For this review, take the finished solid that the model builds, in its own axes (mm). Face numbers are marked on the shaded views. A direction names the side the tool comes from. Coordinates: 2 decimals unless noted, no trailing zeros. Loops run counter-clockwise (first coordinate to the right, second up) from the corner with the lowest first, then second, coordinate; pieces in that order, holes last. Notation, with made-up numbers: M -29,36.25 L -15,36.25 A14 cw -15,53.25 Z; hole C -14.75,73.5 d6. An arc over 180 degrees is marked long. Answer as a JSON object with one key per item and string values. Group by question number.
Item 1: Add section A-A (y = -34.5). State the section outline as (x, z) points, then the cut area to 3 significant figures.
Item 2: Wall thickness on L1, parallel to X at y = -56, z = 38; L2, parallel to Z at x = 57.15, y = -58.75: over which ranges is each line inside the solid? List them lowest first. Write a range as from..to.
Item 3: Tool access review of the marked faces 4, 5 and 6: name each direction out of +Z, -Z, +X, -X, +Y, -Y from which nothing blocks a thin tool from reaching the whole face with its end or side.
Item 4: Insertion check: pin 1 (20.5 mm diameter, centred on x = -71, y = -45, fed in from -Z). The pin has a flat end and moves straight along its axis. Give the tip position at first contact, or say it passes through.
Item 5: Add section B-B (z = 0). State the section outline as (x, y) points (3 decimals), then the cut area to 3 significant figures.
Item 6: Add section C-C (x = -15). State the section outline as (y, z) points (3 decimals), then the cut area to 3 significant figures.
Item 7: Mouldability with a two-part tool opening along X and no side actions: class the marked faces 1, 2 and 3 as +X half, -X half, draft (parallel to the pull), parting line (faces both ways), or undercut.
Item 8: Add section D-D (x = 68). State the section outline as (y, z) points (3 decimals).
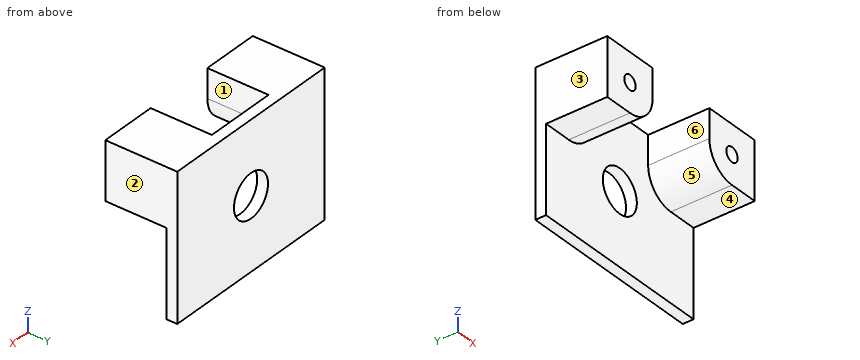
from build123d import *

# Parameters (mm, degrees)
F0_W     = 165.1
F0_H     = 127
F2_DEPTH = 9.525
F3_D     = 38.1
F4_W     = 50.8
F4_H     = 50.8
F5_DEPTH = 63.5
F6_R     = 25.4
F8_D     = 12.7
F8_DEPTH = 12.7
F8_TIP   = 3.8154649308


with BuildPart() as f2:
    # F0 (on Front) → F2 (new body)
    with BuildSketch(Plane.XZ):
        Rectangle(F0_W, F0_H)
    extrude(amount=F2_DEPTH)

    # F3 (through all)
    with Locations(Plane(origin=(0, 0, 0), x_dir=(1, 0, 0), z_dir=(0, 1, 0))):
        with Locations((0, 0)):
            Hole(F3_D / 2)

    # F4 (on Front) → F5 (join)
    with BuildSketch(Plane.XZ):
        with Locations((-57.15, 38.1)):
            Rectangle(F4_W, F4_H)
        with Locations((57.15, 38.1)):
            Rectangle(F4_W, F4_H)
    extrude(amount=F5_DEPTH)

    # F6
    f6_edges = [f2.edges().sort_by_distance(p)[0] for p in [
        (-31.75, -36.5125, 12.7),
        (31.75, -36.5125, 12.7),
    ]]
    fillet(f6_edges, radius=F6_R)

    # F8
    with Locations(Plane.XZ.offset(63.5)):
        with Locations((-57.15, 38.1), (57.15, 38.1)):
            Hole(F8_D / 2, depth=F8_DEPTH)
            with Locations((0, 0, -(F8_DEPTH + F8_TIP / 2))):  # 118° drill point
                Cone(0, F8_D / 2, F8_TIP, mode=Mode.SUBTRACT)


solid = f2.part
From the geometry:
{
 "1": {"outline": "M -82.55,12.7 L -57.15,12.7 A25.4 ccw -31.75,38.1 L -31.75,63.5 L -82.55,63.5 Z; M 31.75,38.1 A25.4 ccw 57.15,12.7 L 82.55,12.7 L 82.55,63.5 L 31.75,63.5 Z", "area": "4,880 mm²"},
 "2": {"L1": "x = -82.55..-63.5, -50.8..-31.75, 31.75..50.8, 63.5..82.55", "L2": "z = 12.7..31.75, 44.45..63.5"},
 "3": {"face 4": "-Z, +X, -X, -Y", "face 5": "-Z, -Y", "face 6": "+Z, -Z, -Y"},
 "4": {"pin 1": "stops at z = 12.7"},
 "5": {"outline": "M -82.55,-9.525 L -19.05,-9.525 L -19.05,0 L -82.55,0 Z; M 19.05,-9.525 L 82.55,-9.525 L 82.55,0 L 19.05,0 Z", "area": "1,210 mm²"},
 "6": {"outline": "M -9.525,-63.5 L 0,-63.5 L 0,-11.743 L -9.525,-11.743 Z; M -9.525,11.743 L 0,11.743 L 0,63.5 L -9.525,63.5 Z", "area": "986 mm²"},
 "7": {"face 1": "undercut", "face 2": "+X half", "face 3": "-X half"},
 "8": {"outline": "M -63.5,12.7 L -9.525,12.7 L -9.525,-63.5 L 0,-63.5 L 0,63.5 L -63.5,63.5 Z"}
}
